Source: CAD feature listing. Evaluate the final solid. Frame: model axes, mm. Face numbers are marked on the shaded views. Give positions to 0.01 mm unless a question says otherwise; leave off trailing zeros. Loops run counter-clockwise (first coordinate to the right, second up) from the corner with the lowest first, then second, coordinate; pieces in that order, holes last. Notation, with made-up numbers: M 1.25,70.25 L 22.25,70.25 A21 cw 22.25,98.25 Z; hole C 83.25,14 d5. An arc over 180 degrees is marked long. Answer in a Markdown table with one row per item.
```python
from build123d import *

# Parameters (mm, degrees)
SKETCH1_W               = 27
SKETCH1_H               = 6
SKETCH1_R               = 1.6
BOSS_EXTRUDE1_DEPTH     = 8
SKETCH3_W               = 27
SKETCH3_H               = 8
BOSS_EXTRUDE2_DEPTH     = 4.5
SKETCH2_R               = 1.6
CUT_EXTRUDE1_DEPTH      = 8.5
CUT_EXTRUDE1_DEPTH_BACK = 4


with BuildPart() as part:
    # Sketch1 → Boss-Extrude1 (new body)
    with BuildSketch(Plane(origin=(0, 0, 0), x_dir=(1, 0, 0), z_dir=(0, 1, 0))):
        with Locations((10, 0)):
            Rectangle(SKETCH1_W, SKETCH1_H)
        Circle(SKETCH1_R, mode=Mode.SUBTRACT)
        with Locations((20, 0)):
            Circle(SKETCH1_R, mode=Mode.SUBTRACT)
    extrude(amount=BOSS_EXTRUDE1_DEPTH)

    # Sketch3 → Boss-Extrude2 (add)
    with BuildSketch(Plane.XY.offset(3)):
        with Locations((10, 4)):
            Rectangle(SKETCH3_W, SKETCH3_H)
    extrude(amount=BOSS_EXTRUDE2_DEPTH)

    # Sketch2 → Cut-Extrude1 (cut, two sides)
    with BuildSketch(Plane.XY) as cut_extrude1_sk:
        with Locations((4.5, 4)):
            Circle(SKETCH2_R)
        with Locations((15.5, 4)):
            Circle(SKETCH2_R)
    extrude(amount=CUT_EXTRUDE1_DEPTH, mode=Mode.SUBTRACT)
    extrude(cut_extrude1_sk.sketch, amount=-CUT_EXTRUDE1_DEPTH_BACK, mode=Mode.SUBTRACT)


solid = part.part
```
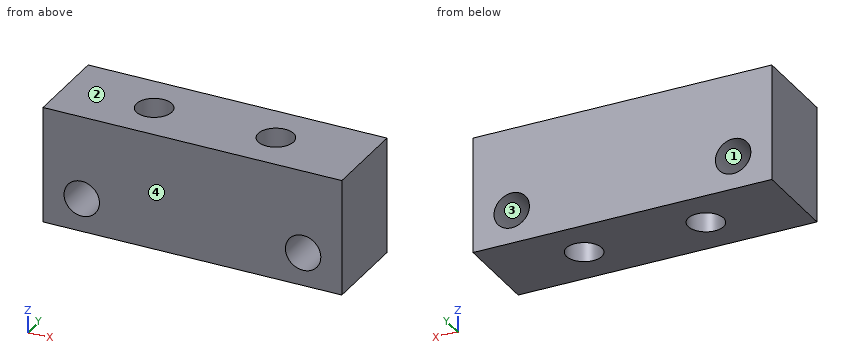
1) Section B-B, the plane x = 20. Return loops of the section in (y, z).
Reply:
| item | result |
|---|---|
| outline | M 0,-3 L 8,-3 L 8,-1.6 L 0,-1.6 Z; M 0,1.6 L 8,1.6 L 8,7.5 L 0,7.5 Z |
2) Pull-direction query (Z, two-part tool) for the marked faces 1, 2, 3 and 4; classes: released by +Z, released by -Z, zero draft, split by the parting line, or undercut.
Reply:
| item | result |
|---|---|
| face 1 | undercut |
| face 2 | released by +Z |
| face 3 | undercut |
| face 4 | zero draft |
3) Section A-A, the plane y = 4. Return loops of the section in (x, z), then the cut area to 3 significant figures.
Reply:
| item | result |
|---|---|
| outline | M -3.5,-3 L 2.9,-3 L 2.9,7.5 L -3.5,7.5 Z; M 6.1,-3 L 13.9,-3 L 13.9,7.5 L 6.1,7.5 Z; M 17.1,-3 L 23.5,-3 L 23.5,7.5 L 17.1,7.5 Z; hole C 0,0 d3.2; hole C 20,0 d3.2 |
| area | 200 mm² |
4) Section C-C, the plane z = 5.5. Return loops of the section in (x, y).
Reply:
| item | result |
|---|---|
| outline | M -3.5,0 L 23.5,0 L 23.5,8 L -3.5,8 Z; hole C 4.5,4 d3.2; hole C 15.5,4 d3.2 |
5) Material intervals for L1, parallel to Y at x = 15.5, z = -1.9; L2, parallel to Z at x = 20, y = 4.75; L3, parallel to X at y = 4.5, z = 0, sorted ascending.
Reply:
| item | result |
|---|---|
| L1 | y = 0 to 2.4, 5.6 to 8 |
| L2 | z = -3 to -1.6, 1.6 to 7.5 |
| L3 | x = -3.5 to -1.6, 1.6 to 2.98, 6.02 to 13.98, 17.02 to 18.4, 21.6 to 23.5 |
6) Section D-D, the plane z = 1. Return loops of the section in (x, y), then the cut area to 3 significant figures.
Reply:
| item | result |
|---|---|
| outline | M -3.5,0 L -1.25,0 L -1.25,8 L -3.5,8 Z; M 1.25,0 L 18.75,0 L 18.75,8 L 1.25,8 Z; M 21.25,0 L 23.5,0 L 23.5,8 L 21.25,8 Z; hole C 4.5,4 d3.2; hole C 15.5,4 d3.2 |
| area | 160 mm² |
